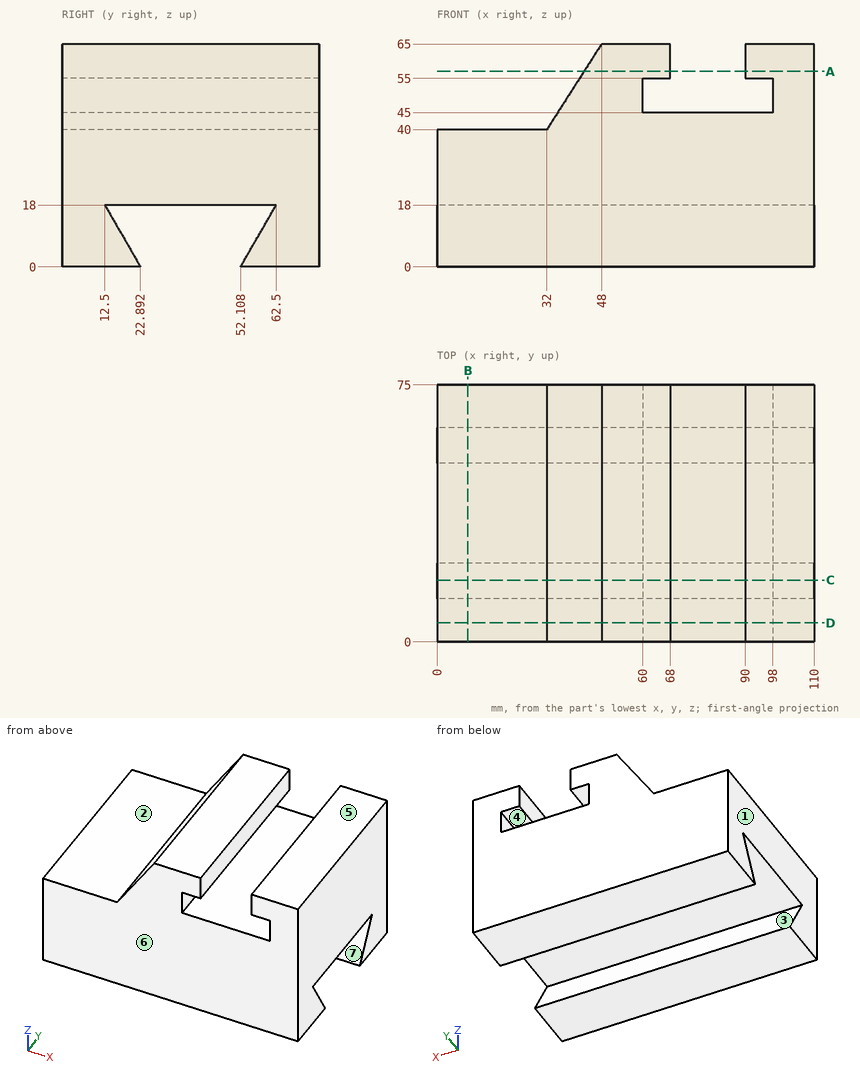
Part print with two shaded views. Sizes in mm from the minimum x, y, z corner. A direction names the side the tool comes from. Round coordinates to 2 decimals unless told otherwise and drop trailing zeros. Write each loop counter-clockwise with the first axis right and the second up, starting at its lowest first coordinate (ties: lowest second). Pieces come first, ordered by that corner, then holes. Notation, with made-up numbers: M 22.5,-20.5 L 67.5,-20.5 A19 cw 67.5,-9.5 Z; hole C -1.75,-24.75 d9. An arc over 180 degrees is marked long. Put each result on its own line as item: value. Start each with the question number.
1) Drill centre lines: probe 1 along Z at (x, y) = (85, 53) (1 decimal); probe 2 along Z at (x, y) = (5, 62) (1 decimal); probe 3 along Z at (x, y) = (25.5, 40.5). Where is each one in solid material? Low to high. Write a range as [from, to].
2) Saw through at A-A, the plane z = 57. Write the cut outline in (x, y), and give its area (3 significant figures).
3) 3-axis set-ups, long thin cutter, end or side, ignore diameter. For the marked faces 1, 2, 3 and 4: which of +Z, -Z, +X, -X, +Y, -Y reach the whole face in a straight line?
4) Saw through at C-C, the plane y = 18. Write the cut outline in (x, z).
5) Saw through at D-D, the plane y = 5.5. Write the cut outline in (x, z), and give its area (3 significant figures).
6) Saw through at B-B, the plane x = 9. Write the cut outline in (y, z).
7) Pull direction Y, two halves, no side cores. Call the marked faces 5, 6 and 7: pulls with the +Y half, pulls with the -Y half, needs draft (parallel to the pull), parting line crosses it, or undercut.
8) Pin check, flat tips, straight feed: pin 1 Ø8 at (y, z) = (32, 52) entering from -X; pin 2 Ø1.5 at (x, y) = (15.5, 49) entering from +Z; pin 3 Ø8 at (y, z) = (46.5, 58) entering from -X. Stop position of each tip, or through.
Resolved:
1. probe 1: [0, 1.5], [18, 45]
1. probe 2: [0, 17.1], [18, 40]
1. probe 3: [18, 40]
2. outline: M 42.88,0 L 68,0 L 68,75 L 42.88,75 Z; M 90,0 L 110,0 L 110,75 L 90,75 Z
2. area: 3,380 mm²
3. face 1: +Z, -Z, -X, +Y, -Y
3. face 2: +Z, -X, +Y, -Y
3. face 3: +X, -X
3. face 4: +Y, -Y
4. outline: M 0,0 L 110,0 L 110,8.47 L 0,8.47 Z; M 0,18 L 110,18 L 110,65 L 90,65 L 90,55 L 98,55 L 98,45 L 60,45 L 60,55 L 68,55 L 68,65 L 48,65 L 32,40 L 0,40 Z
5. outline: M 0,0 L 110,0 L 110,65 L 90,65 L 90,55 L 98,55 L 98,45 L 60,45 L 60,55 L 68,55 L 68,65 L 48,65 L 32,40 L 0,40 Z
5. area: 5,550 mm²
6. outline: M 0,0 L 22.89,0 L 12.5,18 L 62.5,18 L 52.11,0 L 75,0 L 75,40 L 0,40 Z
7. face 5: needs draft
7. face 6: pulls with the -Y half
7. face 7: undercut
8. pin 1: x = 37.12
8. pin 2: z = 40
8. pin 3: x = 40.96
